```python
from build123d import *

# Parameters (mm, degrees)
F2_R    = 5
F3_SIZE = 5
F4_R    = 1.5


with BuildPart() as f1:
    # F0 (on Front) → F1 (revolve)
    with BuildSketch(Plane.XZ):
        Polygon((-60, 0), (0, 0), (0, 15), (-50, 15), (-50, 110), (-77.5635960527, 110), align=None)
    revolve(axis=Axis((0, 0, -4.634299256), (0, 0, -1)))

    # F2
    f2_edges = [f1.edges().sort_by_distance(p)[0] for p in [
        (50, 0, 110),
    ]]
    fillet(f2_edges, radius=F2_R)

    # F3
    f3_edges = [f1.edges().sort_by_distance(p)[0] for p in [
        (77.563596, 0, 110),
    ]]
    chamfer(f3_edges, length=F3_SIZE)

    # F4
    f4_edges = [f1.edges().sort_by_distance(p)[0] for p in [
        (72.563596, 0, 110),
    ]]
    fillet(f4_edges, radius=F4_R)


solid = f1.part
```
Read the model definition and answer for the solid it produces. Units are mm, in the model's axes. Give positions to 0.01 mm unless a question says otherwise; leave off trailing zeros. Order: outer loops, then holes, each group sorted by start corner. A loop starts at its lowest first (then second) coordinate and runs counter-clockwise, first axis right, second up.
(1) For a pull along Y with two mould halves and no side action, classify faces 1 (the flat face through (-16, -53, 110)), 2 (the conical face through (53.99, 49.5, 109.2)), 3 (the cylindrical face through (-47.69, 15.02, 60.63)), 4 (the flat face through (-1, 1, 15)) as released by +Y, released by -Y, zero draft, split by the parting line, or undercut.
(2) Given pin 1 (10 mm diameter, centred on y = -59.5, z = 80.5, fed in from -X); pin 2 (12 mm diameter, centred on x = -56, z = 30, fed in from -Y); pin 3 (10 mm diameter, centred on x = 40, z = 58, fed in from -Y), each flat-ended and moving along its own axis, determine where each tip first touches the part or whether it passes through.
(3) Find section A-A (y = 0). Give the vertices of the cut face in (x, z).
(4) Straight lines are drawn through the part: L1, parallel to Z at x = 20.5, y = 13; L2, parallel to X at y = 2, z = 91.5; L3, parallel to Y at x = 0, z = 62. For each, find the intervals that lie inside material, in ascending order.
(5) Find section D-D (z = 23). Give the vertices of the cut face in (x, y), plus the area to 3 significant figures.
(6) Find section C-C (z = 71.5). Give the vertices of the cut face in (x, y).
Result sheet:
1. face 1: zero draft
1. face 2: split by the parting line
1. face 3: undercut
1. face 4: undercut
2. pin 1: stops at x = -48.47
2. pin 2: stops at y = -41.36
2. pin 3: stops at y = -59.91
3. outline: (-76.78, 105.06) - (-60, 0) - (60, 0) - (76.78, 105.06) - (73.01, 109.47) arc R1.5 ccw to (71.87, 110) - (55, 110) arc R5 ccw to (50, 105) - (50, 15) - (-50, 15) - (-50, 105) arc R5 ccw to (-55, 110) - (-71.87, 110) arc R1.5 ccw to (-73.01, 109.47) - close
4. L1: z = 0 to 15
4. L2: x = -74.58 to -49.96, 49.96 to 74.58
4. L3: y = -69.9 to -50, 50 to 69.9
5. outline: circle Ø127.34 at (0, 0); hole circle Ø100 at (0, 0)
5. area: 4,880 mm2
6. outline: circle Ø142.83 at (0, 0); hole circle Ø100 at (0, 0)
